Could you check a few things on this drawing? It's one solid part, dimensions in mm from its lowest x, y, z. Give positions to 0.01 mm unless a question says otherwise; leave off trailing zeros. Order: outer loops, then holes, each group sorted by start corner. A loop starts at its lowest first (then second) coordinate and runs counter-clockwise, first axis right, second up. Notation, with made-up numbers: (17, 76) - (38, 76) arc R24 cw to (38, 104) - close; hole circle Ø9 at (-28.5, -19). An arc over 180 degrees is marked (long way). One line per question, with ' | ' between items. Start each with the question number.
1. Imagine slicing it at A-A (z = 33.8). Please give me the cut outline in (x, y), and give its area (4 significant figures).
2. I need wall thicknesses on probe 1 along X at (y, z) = (9.75, 7.4). Which ranges of the line are inside material? Lowest first, please. Write a range as from..to.
3. For P1, Ø2.5, axis at x = 1.45, z = 33.8, coming from the -Y side; P2, Ø1.5, axis at x = 12.5, y = 7, coming from the +Z side, each with a flat end and sliding along its axis, tell me the tip position at first contact or that it passes through.
4. Imagine slicing it at B-B (x = 1.45). Please give me the cut outline in (y, z).
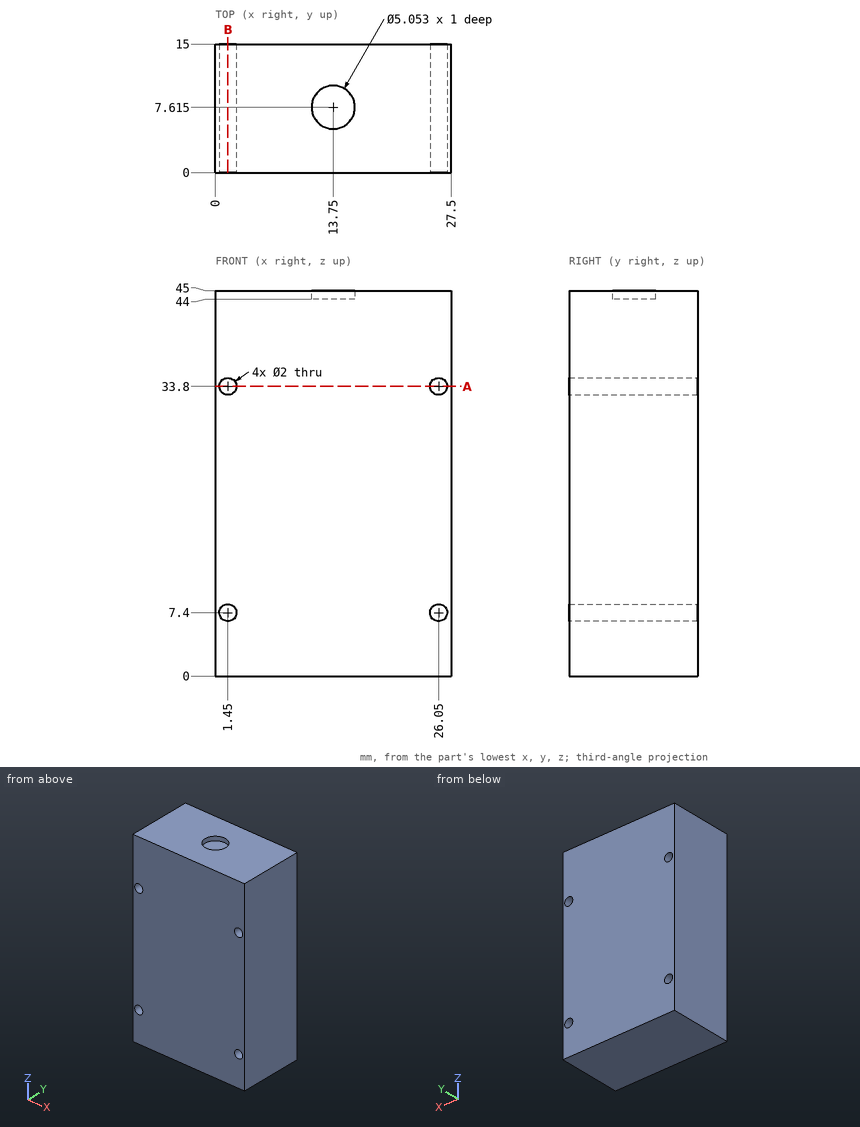
Results found:
1) outline: (0, 0) - (0.45, 0) - (0.45, 15) - (0, 15) - close; (2.45, 0) - (25.05, 0) - (25.05, 15) - (2.45, 15) - close; (27.05, 0) - (27.5, 0) - (27.5, 15) - (27.05, 15) - close | area: 352.5 mm2
2) probe 1: x = 0..0.45, 2.45..25.05, 27.05..27.5
3) P1: stops at y = 0 | P2: stops at z = 44
4) outline: (0, 0) - (15, 0) - (15, 6.4) - (0, 6.4) - close; (0, 8.4) - (15, 8.4) - (15, 32.8) - (0, 32.8) - close; (0, 34.8) - (15, 34.8) - (15, 45) - (0, 45) - close
